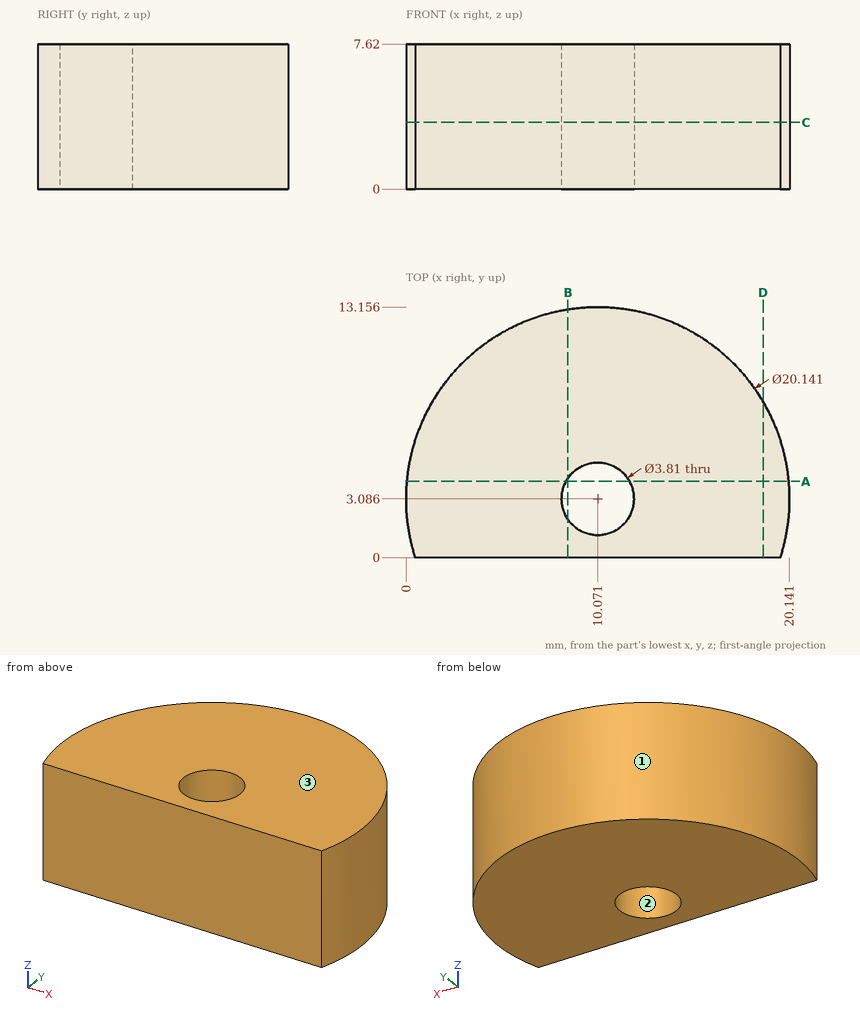
Job drawing, mm, ordinate dimensions from the low corner. One solid piece. Give positions to 0.01 mm unless a question says otherwise; leave off trailing zeros. Loops run counter-clockwise (first coordinate to the right, second up) from the corner with the lowest first, then second, coordinate; pieces in that order, holes last. Notation, with made-up numbers: (-31, 61.5) -> (-10, 61.5) arc R10 ccw to (-10, 80.5) -> close; hole circle Ø6 at (57, -20). An arc over 180 degrees is marked (long way). Write each question's results on one line, items separated by ' | '. Start each with the question number.
Q1. Band-saw the part on C-C on z = 3.5. List the corners of the cut face in (x, y) (1 decimal), plus the area to 3 significant figures.
Q2. Wall check: L1, parallel to X at y = 3, z = 2.25; L2, parallel to Y at x = 10.5, z = 5.5; L3, parallel to X at y = 1.5, z = 3 (1 decimal). Give the ranges that are in metal, low to high.
Q3. Band-saw the part on B-B on x = 8.5. List the corners of the cut face in (y, z).
Q4. Pull direction X, two halves, no side cores. Call the marked faces 1, 2 and 3: +X half, -X half, draft (parallel to the pull), parting line (faces both ways), or undercut.
Q5. Band-saw the part on A-A on y = 4. List the corners of the cut face in (x, z), plus the area to 3 significant figures.
Q6. Band-saw the part on D-D on x = 18.75. List the corners of the cut face in (y, z).
Q7. Pin check, flat tips, straight feed: P1, Ø2, axis at x = 6.5, z = 6.5, coming from the +Y side; P2, Ø4, axis at y = 5.5, z = 5.5, coming from the -X side; P3, Ø2, axis at y = 7, z = 2, coming from the -X side. Stop position of each tip, or through.
Results are:
1) outline: (0.5, 0) -> (19.7, 0) arc R10.1 ccw (long way) to start; hole circle Ø3.8 at (10.1, 3.1) | area: 209 mm²
2) L1: x = 0 to 8.17, 11.97 to 20.14 | L2: y = 0 to 1.23, 4.94 to 13.15 | L3: x = 0.1 to 9, 11.1 to 20
3) outline: (0, 0) -> (2.01, 0) -> (2.01, 7.62) -> (0, 7.62) -> close; (4.16, 0) -> (13.03, 0) -> (13.03, 7.62) -> (4.16, 7.62) -> close
4) face 1: parting line | face 2: undercut | face 3: draft
5) outline: (0.04, 0) -> (8.4, 0) -> (8.4, 7.62) -> (0.04, 7.62) -> close; (11.74, 0) -> (20.1, 0) -> (20.1, 7.62) -> (11.74, 7.62) -> close | area: 127 mm²
6) outline: (0, 0) -> (8.19, 0) -> (8.19, 7.62) -> (0, 7.62) -> close
7) P1: stops at y = 12.82 | P2: stops at x = 0.01 | P3: stops at x = 0.43
